Work out the finished part from the listing and answer in its coordinate system (mm). A direction names the side the tool comes from. Give positions to 0.01 mm unless a question says otherwise; leave off trailing zeros. Order: outer loops, then holes, each group sorted by start corner. A loop starts at its lowest first (then second) coordinate and runs counter-clockwise, first axis right, second up. Notation, with made-up numbers: (25.25, 4) -> (74.25, 4) arc R17 cw to (74.25, 18) -> close; hole circle Ø1 at (-25, 36). An arc over 180 degrees is marked (long way). Use a Markdown table: item, result. Add a question column.
```python
from build123d import *

# Parameters (mm, degrees)
F0_R     = 48.370805
F1_DEPTH = 38.1
F3_DEPTH = 38.1
F4_R     = 35.618168
F5_DEPTH = 66.294


with BuildPart() as f1:
    # F0 (on Top) → F1 (new body)
    with BuildSketch(Plane.XY):
        Circle(F0_R)
    extrude(amount=F1_DEPTH)

    # F2 (on Top) → F3 (join)
    with BuildSketch(Plane.XY):
        Polygon((4.851332, 60.679473), (-4.851332, 60.679473), (-12.616223, 42.146083), (12.616223, 42.146083), align=None)
        Polygon((46.337277, 39.476457), (39.476457, 46.337277), (20.880764, 38.722798), (38.722798, 20.880764), align=None)
        Polygon((60.679473, 4.851332), (42.146083, 12.616223), (42.146083, -12.616223), (60.679473, -4.851332), align=None)
        Polygon((39.476457, -46.337277), (46.337277, -39.476457), (38.722798, -20.880764), (20.880764, -38.722798), align=None)
        Polygon((-4.851332, -60.679473), (4.851332, -60.679473), (12.616223, -42.146083), (-12.616223, -42.146083), align=None)
        Polygon((-46.337277, -39.476457), (-39.476457, -46.337277), (-20.880764, -38.722798), (-38.722798, -20.880764), align=None)
        Polygon((-60.679473, 4.851332), (-60.679473, -4.851332), (-42.146083, -12.616223), (-42.146083, 12.616223), align=None)
        Polygon((-39.476457, 46.337277), (-46.337277, 39.476457), (-38.722798, 20.880764), (-20.880764, 38.722798), align=None)
    extrude(amount=F3_DEPTH)

    # F4 (on face) → F5 (cut)
    with BuildSketch(Plane(origin=(0, 0, 0), x_dir=(1, 0, 0), z_dir=(0, 0, -1))):
        Circle(F4_R)
    extrude(amount=-F5_DEPTH, mode=Mode.SUBTRACT)


solid = f1.part
```
1) Straight lines are drawn through the part: line 1 (X direction, y = 0, z = 16.5); line 2 (X direction, y = -44.5, z = 5). For each, find the intervals that lie inside material, in ascending order.
2) Which of the six approach directions +Z, -Z, +X, -X, +Y, -Y give full straight-line access (tool end or side, diameter ignored) to faces 4 (the cylindrical face through (-18.62, -44.644, 18.783)), 5 (the cylindrical face through (44.644, -18.62, 18.783)), 6 (the flat face through (32.82, 43.61, 18.78)), 7 (the flat face through (-43.534, -32.629, 18.783))?
3) The part is cut by section A-A, the plane x = 0. Determine the outline of the cut face in (y, z).
4) The part is cut by section D-D, the plane x = 52.5. Determine the outline of the cut face in (y, z), then the cut area to 3 significant figures.
5) Determine the mould class of faces 1 (the flat face through (32.629, -43.534, 18.783)), 2 (the flat face through (7.71, 53.86, 18.78)), 3 (the flat face through (-42.955, -42.859, 18.783)) for opening direction X: released by +X, released by -X, zero draft, split by the parting line, or undercut.
6) Flat-ended cylindrical pins translate along their axes: pin 1 (2 mm diameter, centred on x = 8.5, z = 12.5, fed in from +Y); pin 2 (5 mm diameter, centred on x = -10.5, z = 32.5, fed in from +Y); pin 3 (12 mm diameter, centred on x = -37.5, z = 9, fed in from -Y). Find the tip coordinate at first contact, or state that the pin passes through.
A:
| question | item | result |
|---|---|---|
| 1 | line 1 | -60.68 to -35.62, 35.62 to 60.68 |
| 1 | line 2 | -41.31 to -34.99, -18.96 to 18.96, 34.99 to 41.31 |
| 2 | face 4 | +Z, -Z, -Y |
| 2 | face 5 | +Z, -Z, +X |
| 2 | face 6 | +Z, -Z, +Y |
| 2 | face 7 | +Z, -Z, -X |
| 3 | outline | (-60.68, 0) -> (-35.62, 0) -> (-35.62, 38.1) -> (-60.68, 38.1) -> close; (35.62, 0) -> (60.68, 0) -> (60.68, 38.1) -> (35.62, 38.1) -> close |
| 4 | outline | (-8.28, 0) -> (8.28, 0) -> (8.28, 38.1) -> (-8.28, 38.1) -> close |
| 4 | area | 631 mm^2 |
| 5 | face 1 | undercut |
| 5 | face 2 | released by +X |
| 5 | face 3 | released by -X |
| 6 | pin 1 | y = 54.36 |
| 6 | pin 2 | y = 53.16 |
| 6 | pin 3 | y = -46.34 |
